Read the model definition and answer for the solid it produces. Units are mm, in the model's axes. Coordinates: 2 decimals unless noted, no trailing zeros. Loops run counter-clockwise (first coordinate to the right, second up) from the corner with the lowest first, then second, coordinate; pieces in that order, holes last. Notation, with made-up numbers: M 8,74.25 L 13,74.25 A27 cw 13,108.25 Z; hole C 3,-14 d7. An arc over 180 degrees is marked long. Put each result on its own line as item: value.
from build123d import *

# Parameters (mm, degrees)
BOSS_EXTRUDE2_DEPTH = 10
SKETCH4_W           = 20
SKETCH4_H           = 20
CUT_EXTRUDE1_DEPTH  = 10
SKETCH5_W           = 22
SKETCH5_H           = 22
CUT_EXTRUDE2_DEPTH  = 11
SKETCH6_R           = 150
CUT_EXTRUDE3_DEPTH  = 11


with BuildPart() as part:
    # Sketch1 → Boss-Extrude2 (new body)
    with BuildSketch(Plane(origin=(0, 0, 0), x_dir=(1, 0, 0), z_dir=(0, 1, 0))):
        Polygon((0, 0), (246.777636447, 0), (246.777636447, 660.361240582), (-103.222363553, 660.361240582), (-100.13363069, 640.601186703), (-200.677997122, 489.475620291), (-200.677997122, 330.180620291), (-200.677997122, 170.885620291), (0, 20), align=None)
    extrude(amount=BOSS_EXTRUDE2_DEPTH)

    # Sketch4 → Cut-Extrude1 (cut)
    with BuildSketch(Plane(origin=(0, 10, 0), x_dir=(1, 0, 0), z_dir=(0, 1, 0))):
        with Locations((-10, 348.38)):
            Rectangle(SKETCH4_W, SKETCH4_H)
    extrude(amount=-CUT_EXTRUDE1_DEPTH, mode=Mode.SUBTRACT)

    # Sketch5 → Cut-Extrude2 (cut, through all)
    with BuildSketch(Plane.XZ):
        with Locations((235.777636447, -649.361240582)):
            Rectangle(SKETCH5_W, SKETCH5_H)
        with Locations((235.777636447, -11)):
            Rectangle(SKETCH5_W, SKETCH5_H)
    extrude(amount=-CUT_EXTRUDE2_DEPTH, mode=Mode.SUBTRACT)

    # Sketch6 → Cut-Extrude3 (cut, through all)
    with BuildSketch(Plane(origin=(0, 10, 0), x_dir=(1, 0, 0), z_dir=(0, 1, 0))):
        with Locations((32.340951638, 229.684080555)):
            Circle(SKETCH6_R)
    extrude(amount=-CUT_EXTRUDE3_DEPTH, mode=Mode.SUBTRACT)


solid = part.part
1) Find section D-D, the plane z = -551. Write down the section's boundary in (x, y), plus the area to 3 significant figures.
Answer list:
outline: M -159.75,0 L 246.78,0 L 246.78,10 L -159.75,10 Z
area: 4,070 mm^2
2) Given pin 1 Ø6 at (x, z) = (191.5, -369) entering from -Y; pin 2 Ø3 at (y, z) = (6, -16) entering from +X, each flat-ended and moving along its own axis, determine where each tip first touches the part or whether it passes through.
Answer list:
pin 1: stops at y = 0
pin 2: stops at x = 224.78
3) Find section C-C, the plane y = 4. Write down the section's boundary in (x, z).
Answer list:
outline: M -200.68,-489.48 L -100.13,-640.6 L -103.22,-660.36 L 224.78,-660.36 L 224.78,-638.36 L 246.78,-638.36 L 246.78,-22 L 224.78,-22 L 224.78,0 L 0,0 L 0,-20 L -200.68,-170.89 Z; hole C 32.34,-229.68 d300
4) Find section A-A, the plane x = -27. Write down the section's boundary in (y, z), plus the area to 3 significant figures.
Answer list:
outline: M 0,-660.36 L 10,-660.36 L 10,-367.45 L 0,-367.45 Z; M 0,-91.92 L 10,-91.92 L 10,-40.3 L 0,-40.3 Z
area: 3,450 mm^2
5) Straight lines are drawn through the part: line 1 (Z direction, x = 15.5, y = 3.25); line 2 (Z direction, x = 6.5, y = 4.25); line 3 (X direction, y = 1.5, z = -98). For each, find the intervals that lie inside material, in ascending order. Write a range as [from, to].
Answer list:
line 1: z = [-660.36, -378.74], [-80.63, 0]
line 2: z = [-660.36, -377.44], [-81.93, 0]
line 3: x = [-103.74, -39.49], [104.17, 246.78]
6) Determine the mould class of faces 1 (the cylindrical face through (-0.18, 5.07, -83.25)), 2 (the flat face through (-149.7, 4.9, -566.1)), 3 (the flat face through (20, 0, -408)) for opening direction X: released by +X, released by -X, zero draft, split by the parting line, or undercut.
Answer list:
face 1: undercut
face 2: released by -X
face 3: zero draft
7) Find section B-B, the plane z = -113.5. Write down the section's boundary in (x, y).
Answer list:
outline: M -124.36,0 L -62.53,0 L -62.53,10 L -124.36,10 Z; M 127.22,0 L 246.78,0 L 246.78,10 L 127.22,10 Z
